from build123d import *

# Parameters (mm, degrees)
BOSS_EXTRUDE1_DEPTH        = 1.016
F_2_9_2_9_DIAMETER_HOLE1_D = 2.9
CHAMFER1_SIZE              = 0.7
SKETCH4_R                  = 6
CUT_EXTRUDE1_DEPTH         = 112.324431389
CUT_EXTRUDE2_DEPTH         = 112.324431389


with BuildPart() as part:
    # Sketch1 → Boss-Extrude1 (new, symmetric)
    with BuildSketch(Plane(origin=(0, 0, 0), x_dir=(1, 0, 0), z_dir=(0, 1, 0))):
        with BuildLine():
            Line((-82, -58), (82, -58))
            ThreePointArc((82, -58), (91.192388155, -54.192388155), (95, -45))
            Line((95, -45), (95, 45))
            ThreePointArc((95, 45), (91.192388155, 54.192388155), (82, 58))
            Line((82, 58), (-82, 58))
            ThreePointArc((-82, 58), (-91.192388155, 54.192388155), (-95, 45))
            Line((-95, 45), (-95, -45))
            ThreePointArc((-95, -45), (-91.192388155, -54.192388155), (-82, -58))
        make_face()
    extrude(amount=BOSS_EXTRUDE1_DEPTH, both=True)

    # Ø2.9 (2.9) Diameter Hole1 (through all)
    with Locations(Plane(origin=(0, 1.016, 0), x_dir=(1, 0, 0), z_dir=(0, 1, 0))):
        with Locations((-88, -51), (-88, 51), (88, -51), (88, 51)):
            Hole(F_2_9_2_9_DIAMETER_HOLE1_D / 2)

    # Chamfer1
    chamfer1_edges = [part.edges().sort_by_distance(p)[0] for p in [
        (89.45, 1.016, -51),
        (89.45, -1.016, -51),
        (89.45, 1.016, 51),
        (-86.55, 1.016, -51),
        (-86.55, 1.016, 51),
    ]]
    chamfer(chamfer1_edges, length=CHAMFER1_SIZE)

    # Sketch4 → Cut-Extrude1 (cut, through all)
    with BuildSketch(Plane(origin=(0, 1.016, 0), x_dir=(1, 0, 0), z_dir=(0, 1, 0))):
        with Locations(Location((-13.1, 43.4, 0), (0, 0, 270))):
            Circle(SKETCH4_R)
    extrude(amount=-CUT_EXTRUDE1_DEPTH, mode=Mode.SUBTRACT)

    # Sketch5 → Cut-Extrude2 (cut, through all)
    with BuildSketch(Plane(origin=(0, 1.016, 0), x_dir=(1, 0, 0), z_dir=(0, 1, 0))):
        with BuildLine():
            Line((1.9, 46.4), (26.9, 46.4))
            ThreePointArc((26.9, 46.4), (29.9, 43.4), (26.9, 40.4))
            Line((26.9, 40.4), (1.9, 40.4))
            ThreePointArc((1.9, 40.4), (-1.1, 43.4), (1.9, 46.4))
        make_face()
    extrude(amount=-CUT_EXTRUDE2_DEPTH, mode=Mode.SUBTRACT)


solid = part.part
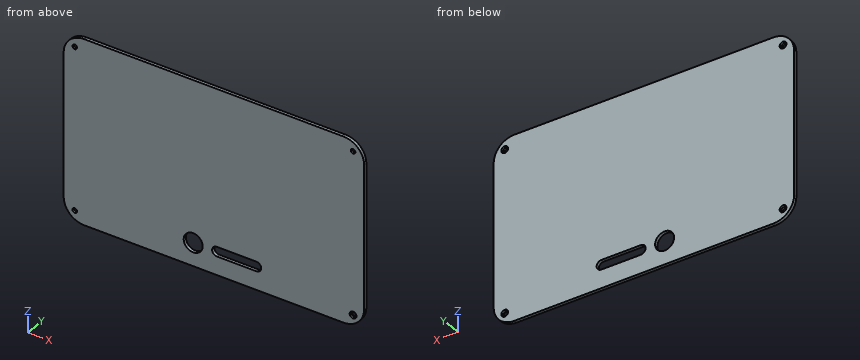
Build history of the part. All positions in model axes, mm. Coordinates: 2 decimals unless noted, no trailing zeros. Write each loop counter-clockwise with the first axis right and the second up, starting at its lowest first coordinate (ties: lowest second). Pieces come first, ordered by that corner, then holes.
(1) Cut at A-A on x = -13.1. List the corners of the cut face in (y, z).
(2) Drill centre lines: line 1 (X direction, y = -0.4, z = -43.4); line 2 (Z direction, x = 12.5, y = 0.5); line 3 (Z direction, x = 88, y = -0.4). Where is each one in solid material? Low to high.
(3) Pin check, flat tips, straight feed: pin 1 Ø1.7 at (x, z) = (-88, 51) entering from -Y; pin 2 Ø3.5 at (x, z) = (88, -51) entering from +Y. Stop position of each tip, or through.
Working result:
1. outline: (-1.02, -58) - (1.02, -58) - (1.02, -49.4) - (-1.02, -49.4) - close; (-1.02, -37.4) - (1.02, -37.4) - (1.02, 58) - (-1.02, 58) - close
2. line 1: x = -95 to -19.1, -7.1 to -1.1, 29.9 to 95
2. line 2: z = -58 to -46.4, -40.4 to 58
2. line 3: z = -56.53 to -52.53, -49.47 to 49.55, 52.45 to 56.53
3. pin 1: passes through
3. pin 2: stops at y = 0.62
